```python
from build123d import *

# Parameters (mm, degrees)
SKETCH1_W           = 8.6
SKETCH1_H           = 4.5
BOSS_EXTRUDE1_DEPTH = 4.7
SKETCH2_W           = 4.1
SKETCH2_H           = 2.5
CUT_EXTRUDE1_DEPTH  = 0.5
BOSS_EXTRUDE2_DEPTH = 0.4
SKETCH4_R           = 0.25
BOSS_EXTRUDE3_DEPTH = 3
SKETCH5_W           = 2
SKETCH5_H           = 2
BOSS_EXTRUDE4_DEPTH = 4.6
CUT_EXTRUDE2_REACH  = 8.7
FILLET2_R           = 0.1


with BuildPart() as part:
    # Sketch1 → Boss-Extrude1 (new body)
    with BuildSketch(Plane.XY):
        Rectangle(SKETCH1_W, SKETCH1_H)
    extrude(amount=BOSS_EXTRUDE1_DEPTH)

    # Sketch2 → Cut-Extrude1 (cut)
    with BuildSketch(Plane.XZ.offset(2.25)):
        with Locations((0, 2.7)):
            Rectangle(SKETCH2_W, SKETCH2_H)
    extrude(amount=-CUT_EXTRUDE1_DEPTH, mode=Mode.SUBTRACT)

    # Sketch3 → Boss-Extrude2 (add)
    with BuildSketch(Plane(origin=(4.3, 0, 0), x_dir=(0, 0, -1), z_dir=(1, 0, 0))):
        with BuildLine():
            Line((0, 0.6), (0, -0.6))
            Line((0, -0.6), (2.2, -0.6))
            ThreePointArc((2.2, -0.6), (2.8, 0), (2.2, 0.6))
            Line((2.2, 0.6), (0, 0.6))
        make_face()
    boss_extrude2 = extrude(amount=-BOSS_EXTRUDE2_DEPTH)

    # Mirror1: Boss-Extrude2 across plane
    add(boss_extrude2.mirror(Plane(origin=(0, 0, 0), x_dir=(0, 0, 1), z_dir=(1, 0, 0))))

    # Sketch4 → Boss-Extrude3 (add)
    with BuildSketch(Plane(origin=(0, 0, 0), x_dir=(-1, 0, 0), z_dir=(0, 0, -1))):
        with Locations((2, 0)):
            Circle(SKETCH4_R)
        Circle(SKETCH4_R)
        with Locations((-2, 0)):
            Circle(SKETCH4_R)
    extrude(amount=BOSS_EXTRUDE3_DEPTH)

    # Sketch5 → Boss-Extrude4 (add)
    with BuildSketch(Plane.XZ.offset(1.75)):
        with Locations((-1, 2.7)):
            Rectangle(SKETCH5_W, SKETCH5_H)
    extrude(amount=BOSS_EXTRUDE4_DEPTH)

    # Sketch6 → Cut-Extrude2 (cut, up to next)
    with BuildSketch(Plane.XY.offset(3.7), mode=Mode.PRIVATE) as cut_extrude2_sk1:
        Polygon((-1, -5.975), (-1.375, -6.35), (-0.625, -6.35), align=None)
    cut_extrude2_tool1 = extrude(cut_extrude2_sk1.sketch, amount=-CUT_EXTRUDE2_REACH, mode=Mode.PRIVATE) & part.part
    add(cut_extrude2_tool1.solids().sort_by_distance((-1, -6.225, 3.7))[0], mode=Mode.SUBTRACT)

    # Fillet2
    fillet2_edges = [part.edges().sort_by_distance(p)[0] for p in [
        (4.3, 0, 4.7),
        (0, 2.25, 4.7),
        (-4.3, 0, 4.7),
        (-1.75, 0, -3),
        (0.25, 0, -3),
        (2.25, 0, -3),
        (0, -2.25, 4.7),
    ]]
    fillet(fillet2_edges, radius=FILLET2_R)


solid = part.part
```
Work out the finished part from the listing and answer in its coordinate system (mm). A direction names the side the tool comes from. Coordinates: 2 decimals unless noted, no trailing zeros. Loops run counter-clockwise (first coordinate to the right, second up) from the corner with the lowest first, then second, coordinate; pieces in that order, holes last. Notation, with made-up numbers: M 73,1.5 L 103,1.5 A23 cw 103,11.5 Z; hole C 4,-4.75 d9. An arc over 180 degrees is marked long. Use CSV: the item, a comma, the result in double quotes. Start each with the question number.
(1) Find section B-B, the plane y = -2. Give the vertices of the cut face in (x, z), then the cut area to 3 significant figures.
(2) Find section C-C, the plane y = 0. Give the vertices of the cut face in (x, z).
(3) For faces 1 (the face through (0, 1, 0)), 2 (the face through (3.9, 0, -1)), 3 (the face through (0, 0, 4.7)), determine the directions among +Z, -Z, +X, -X, +Y, -Y from which every point of the face is accessible in a straight line to the end or side of a thin tool.
(4) For a pull along X with two mould halves and no side action, classify faces 4 (the face through (1, -1.75, 3)), 5 (the face through (-4.3, 0, 2)), 6 (the face through (0, 2.25, 2)) as +X half, -X half, draft (parallel to the pull), parting line (faces both ways), or undercut.
(5) Find section A-A, the plane z = -1.75. Give the vertices of the cut face in (x, y).
(6) Find section D-D, the plane x = 2.5. Give the vertices of the cut face in (y, z).
(7) Consider line 1 (Y direction, x = 2.25, z = 2); line 2 (Z direction, x = -1, y = 1.25); line 3 (X direction, y = -3, z = 2.75). Determine where each line is inside the solid, lowest interval first.
(8) Given pin 1 Ø0.6 at (x, y) = (-1.5, -4) entering from -Z; pin 2 Ø0.6 at (y, z) = (-4, 3) entering from +X; pin 3 Ø1.5 at (x, z) = (-2.5, -2) entering from +Y, each flat-ended and moving along its own axis, determine where each tip first touches the part or whether it passes through.
Recorded:
1,outline,"M -4.3,0 L 4.3,0 L 4.3,4.6 A0.1 ccw 4.2,4.7 L -4.2,4.7 A0.1 ccw -4.3,4.6 Z; M -2,1.7 L 0,1.7 L 0,3.7 L -2,3.7 Z; hole M -2.05,1.45 L 2.05,1.45 L 2.05,3.95 L -2.05,3.95 Z"
1,area,"34.2 mm^2"
2,outline,"M -4.3,-2.8 L -3.9,-2.8 L -3.9,0 L -2.25,0 L -2.25,-2.9 A0.1 ccw -2.15,-3 L -1.85,-3 A0.1 ccw -1.75,-2.9 L -1.75,0 L -0.25,0 L -0.25,-2.9 A0.1 ccw -0.15,-3 L 0.15,-3 A0.1 ccw 0.25,-2.9 L 0.25,0 L 1.75,0 L 1.75,-2.9 A0.1 ccw 1.85,-3 L 2.15,-3 A0.1 ccw 2.25,-2.9 L 2.25,0 L 3.9,0 L 3.9,-2.8 L 4.3,-2.8 L 4.3,4.6 A0.1 ccw 4.2,4.7 L -4.2,4.7 A0.1 ccw -4.3,4.6 Z"
3,face 1,"-Z"
3,face 2,"-Z, +Y, -Y"
3,face 3,"+Z, +X, -X, +Y, -Y"
4,face 4,"undercut"
4,face 5,"-X half"
4,face 6,"draft"
5,outline,"M -4.3,-0.6 L -3.9,-0.6 L -3.9,0.6 L -4.3,0.6 Z; C -2,0 d0.5; C 0,0 d0.5; C 2,0 d0.5; M 3.9,-0.6 L 4.3,-0.6 L 4.3,0.6 L 3.9,0.6 Z"
6,outline,"M -2.25,0 L 2.25,0 L 2.25,4.6 A0.1 ccw 2.15,4.7 L -2.15,4.7 A0.1 ccw -2.25,4.6 Z"
7,line 1,"y = -2.25 to 2.25"
7,line 2,"z = 0 to 4.7"
7,line 3,"x = -2 to 0"
8,pin 1,"stops at z = 1.7"
8,pin 2,"stops at x = 0"
8,pin 3,"stops at y = 0.25"
